Model file for the job. Use its own axes, mm. Face numbers are marked on the shaded views. A direction names the side the tool comes from. Round coordinates to 2 decimals unless told otherwise and drop trailing zeros. Order: outer loops, then holes, each group sorted by start corner. A loop starts at its lowest first (then second) coordinate and runs counter-clockwise, first axis right, second up. Notation, with made-up numbers: (47, -14.75) -> (105, -14.75) arc R22 cw to (105, 16.25) -> close; hole circle Ø9 at (15, 20). An arc over 180 degrees is marked (long way). Use CSV: the item, a comma, the result in double quotes.
```python
from build123d import *

# Parameters (mm, degrees)
SKETCH1_W           = 15
SKETCH1_H           = 15
BOSS_EXTRUDE1_DEPTH = 93
SKETCH2_R           = 3
BOSS_EXTRUDE2_DEPTH = 7
FILLET1_R           = 2


with BuildPart() as part:
    # Sketch1 → Boss-Extrude1 (new body)
    with BuildSketch(Plane(origin=(0, 0, 0), x_dir=(1, 0, 0), z_dir=(0, 1, 0))):
        Rectangle(SKETCH1_W, SKETCH1_H)
    extrude(amount=BOSS_EXTRUDE1_DEPTH)

    # Sketch2 → Boss-Extrude2 (add)
    with BuildSketch(Plane(origin=(0, 93, 0), x_dir=(1, 0, 0), z_dir=(0, 1, 0))):
        with Locations(Location((1.5, -2.5, 0), (0, 0, 90))):
            Circle(SKETCH2_R)
    extrude(amount=BOSS_EXTRUDE2_DEPTH)

    # Fillet1
    fillet1_edges = [part.edges().sort_by_distance(p)[0] for p in [
        (7.5, 46.5, 7.5),
    ]]
    fillet(fillet1_edges, radius=FILLET1_R)


solid = part.part
```
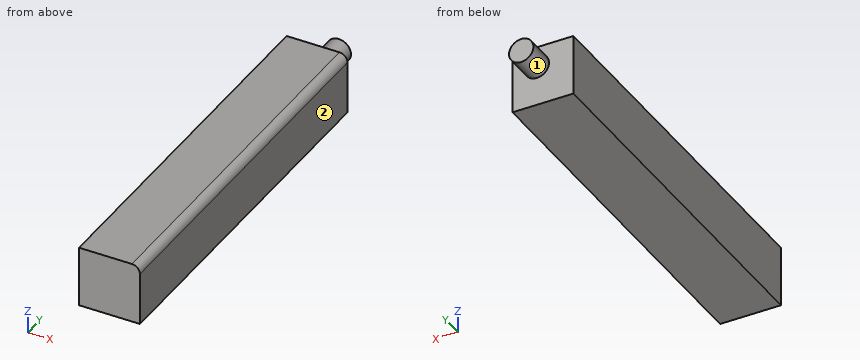
Q1. Which spindle directions (+Z, -Z, +X, -X, +Y, -Y) get a long thin tool onto all of the face, cutting with end or side? Do the marked faces 1 and 2. Say none if no direction does.
From the geometry:
face 1,"+Y"
face 2,"+Z, -Z, +X, +Y, -Y"
Q2. Probe line 1 along Y through (x, z) = (-5.5, 2.25); line 2 along Z through (x, y) = (5.75, 77.5); line 3 along Z through (x, y) = (6.5, 25). List the from-to ranges inside material, lowest first.
From the geometry:
line 1,"y = 0 to 93"
line 2,"z = -7.5 to 7.48"
line 3,"z = -7.5 to 7.23"
Q3. Cut at A-A (z = 2.5). Give the cut face in (x, y).
From the geometry:
outline,"(-7.5, 0) -> (7.5, 0) -> (7.5, 93) -> (4.5, 93) -> (4.5, 100) -> (-1.5, 100) -> (-1.5, 93) -> (-7.5, 93) -> close"
Q4. Cut at B-B (x = 1.5). Give the cut face in (y, z), plus the area to 3 significant figures.
From the geometry:
outline,"(0, -7.5) -> (93, -7.5) -> (93, -0.5) -> (100, -0.5) -> (100, 5.5) -> (93, 5.5) -> (93, 7.5) -> (0, 7.5) -> close"
area,"1,440 mm²"
Q5. Pin check, flat tip, straight feed: pin 1 (3 mm diameter, centred on x = -3, z = -3.5, fed in from +Y). Stop position of the tip, or through.
From the geometry:
pin 1,"stops at y = 93"
